Verification items for the finished model (mm, model axes). Face numbers are marked on the shaded views. A direction names the side the tool comes from. Round coordinates to 2 decimals unless told otherwise and drop trailing zeros. Write each loop counter-clockwise with the first axis right and the second up, starting at its lowest first coordinate (ties: lowest second). Pieces come first, ordered by that corner, then holes. Notation, with made-up numbers: (57, 87.25) - (109, 87.25) arc R33 cw to (109, 115.25) - close; hole circle Ø4 at (19, -5.5). An arc over 180 degrees is marked (long way). Answer as a JSON object with one key per item and string values. Group by question number.
1) Section check A-A (y = 30.5). Enter the section's corners in (x, z), then the cut area to 3 significant figures.
2) Section check D-D (x = -34.5). Enter the section's corners in (y, z).
3) Section check B-B (x = 8.5). Enter the section's corners in (y, z), then the cut area to 3 significant figures.
4) Section check C-C (z = 19). Enter the section's corners in (x, y), then the cut area to 3 significant figures.
5) Go/stop test with flat-tipped pins: pin 1 Ø4 at (y, z) = (124, 94) entering from +X; pin 2 Ø6.5 at (x, z) = (30, 95.5) entering from -Y; pin 3 Ø1.8 at (x, z) = (-25, 44.5) entering from +Y. Record where each tip stops, or that it passes through.
6) Mould release check, pull along X, two halves, no side actions. Record for the marked faces 4, 5 and 6: +X half, -X half, draft (parallel to the pull), parting line (faces both ways), or undercut.
7) Thickness scan on line 1 (Y direction, x = 19.5, z = 26.5); line 2 (Y direction, x = 46, z = 22); line 3 (Z direction, x = 13.5, y = 10). Record the ranges inside material, lowest first.
8) Set-up check for the marked faces 1, 2 and 3: record each of +Z, -Z, +X, -X, +Y, -Y from which the full face is reachable in a straight line by a thin tool's end or side.
Autodesk Inventor part; units mm, degrees
ref_plane "Work Plane1" through (-48, 65, 2) normal (0, -1, 0) x (1, 0, 0)
ref_plane "Work Plane3" through (-48, 165, 5) normal (0, 1, 0) x (1, 0, 0)
ref_plane "Work Plane2" through (-48, 165, 5) normal (0, 1, 0) x (1, 0, 0)
sketch "Sketch2" plane through (0, 0, 0) normal (0, 0, 1) x (1, 0, 0)
  line L0 (0, 0) -> (70, 0)
  line L1 (70, 0) -> (70, 165)
  line L2 (70, 165) -> (0, 165)
  line L3 (0, 165) -> (0, 0)
  dimension "d0" = 165
  dimension "d1" = 70
extrude "Extrusion1" add sketch "Sketch2" along normal blind 90
sketch "Sketch6" plane through (0, 0, 0) normal (-1, 0, 0) x (0, 0, 1)
  line L0 (90, 0) -> (90, 165)
  line L1 (0, 0) -> (0, 165)
  line L2 (90, 165) -> (0, 165)
  line L3 (0, 165) -> (0, 65)
  line L4 (0, 65) -> (90, 65)
  line L5 (90, 65) -> (90, 165)
  dimension "d8" = 100
extrude "Extrusion3" add sketch "Sketch6" along normal blind 50
sketch "Sketch7" plane through (0, 65, 0) normal (0, -1, 0) x (1, 0, 0)
  line L0 (70, 90) -> (-50, 90)
  line L1 (0, 0) -> (0, 90)
  line L2 (-50, 90) -> (0, 90)
  line L3 (0, 90) -> (0, 38)
  line L4 (0, 38) -> (-50, 38)
  line L5 (-50, 38) -> (-50, 90)
  dimension "d11" = 52
extrude "Extrusion4" add sketch "Sketch7" along normal blind 75
sketch "Sketch8" plane through (0, 65, 38) normal (0, 0, -1) x (-1, 0, 0)
  line L0 (0, 0) -> (50, 0)
  line L1 (50, 0) -> (29, 0)
  line L2 (29, 0) -> (29, -45)
  line L3 (29, -45) -> (50, -45)
  line L4 (50, -45) -> (50, 0)
  point P0 (0, -65)
  point P1 (29, 0)
  dimension "d14" = 21
  dimension "d15" = 45
extrude "Extrusion5" add sketch "Sketch8" along normal blind 25
sketch "Sketch9" plane through (0, 0, 90) normal (0, 0, 1) x (1, 0, 0)
  line L0 (70, 165) -> (-50, 165)
  line L1 (-50, 165) -> (70, 165)
  line L2 (70, 165) -> (10, 165)
  line L3 (10, 70) -> (57.5, 70)
  line L4 (57.5, 70) -> (-37.5, 70)
  line L5 (-37.5, 70) -> (-37.5, 165)
  line L6 (57.5, 70) -> (57.5, 165)
  point P0 (0, 0)
  dimension "d20" = 95
  dimension "d21" = 95
extrude "Extrusion6" add sketch "Sketch9" along normal blind 8
ref_plane "Work Plane1" through (-48, 65, 2) normal (0, -1, 0) x (1, 0, 0)
sketch "Sketch10" plane through (-48, 65, 2) normal (0, -1, 0) x (1, 0, 0)
  line L0 (21, 34) -> (46, 34)
  line L1 (33.5, 34) -> (33.5, 0)
  line L2 (46, 0) -> (0, 0)
  circle A0 centre (33.5, 17) radius 12.5
  point P0 (48, -2)
extrude "Extrusion7" add sketch "Sketch10" along normal blind 70
ref_plane "Work Plane3" through (-48, 165, 5) normal (0, 1, 0) x (1, 0, 0)
sketch "Sketch11" plane through (-48, 165, 5) normal (0, 1, 0) x (1, 0, 0)
  line L0 (113, 0) -> (113, -80)
  line L1 (0, -80) -> (0, 0)
  circle A0 centre (56.5, -40) radius 21
  point P0 (48, 5)
  dimension "d29" = 42
extrude "Extrusion8" add sketch "Sketch11" along normal blind 6
ref_plane "Work Plane2" through (-48, 165, 5) normal (0, 1, 0) x (1, 0, 0)
sketch "Sketch12" plane through (-48, 165, 5) normal (0, 1, 0) x (1, 0, 0)
  circle A0 centre (56.5, -40) radius 21
  line L0 (35.5, -40) -> (26.5, -40)
  circle A1 centre (23.5, -40) radius 3
  point P0 (48, 5)
  dimension "d32" = 9
extrude "Extrusion9" add sketch "Sketch12" along normal blind 7 contours A1
sketch "Sketch13" plane through (8.5, 171, 45) normal (0, 1, 0) x (1, 0, 0)
  circle A0 centre (0, 0) radius 22.5
  arc A1 (21.4111, -6.9148) -> (21.4111, 6.9148) centre (22.5, 0) ccw
  point P0 (-8.5, 45)
  dimension "d37" = 45
  dimension "d38" = 14
extrude "Extrusion10" add sketch "Sketch13" along normal mid plane 6 contours A0
extrude "Extrusion11" add sketch "Sketch13" along normal blind 2 contours A0 A1
fillet "Fillet3" radius 10 4 edges at (-50, 115, 0) (70, 82.5, 0) (70, 82.5, 90) (-50, 77.5, 90)
properties part number "windshield washer"
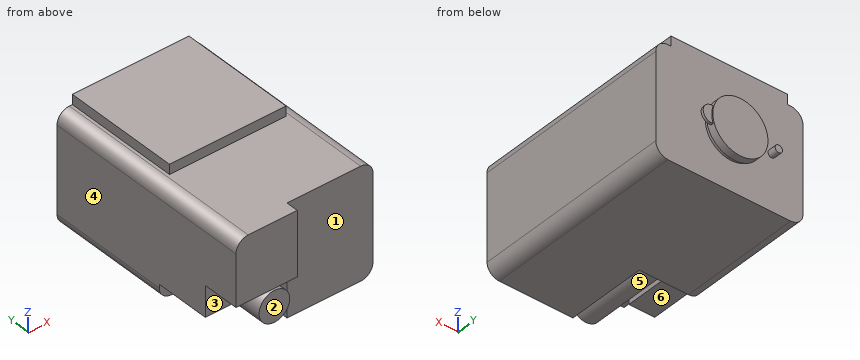
Returned:
{
 "1": {"outline": "(-50, 13) - (-29, 13) - (-29, 38) - (0, 38) - (0, 0) - (60, 0) arc R10 ccw to (70, 10) - (70, 80) arc R10 ccw to (60, 90) - (-40, 90) arc R10 ccw to (-50, 80) - close; circle Ø25 at (-14.5, 19)", "area": "9,850 mm2"},
 "2": {"outline": "(-10, 38) - (20, 38) - (20, 13) - (65, 13) - (65, 0) - (165, 0) - (165, 98) - (70, 98) - (70, 90) - (-10, 90) - close"},
 "3": {"outline": "(0, 0) - (165, 0) - (165, 24) - (168, 24) - (168, 22.5) - (174, 22.5) - (174, 67.5) - (168, 67.5) - (168, 66) - (165, 66) - (165, 98) - (70, 98) - (70, 90) - (0, 90) - close", "area": "16,000 mm2"},
 "4": {"outline": "(-50, 20) - (-29, 20) - (-29, 65) - (-27, 65) - (-27, -5) - (-2, -5) - (-2, 65) - (0, 65) - (0, 0) - (70, 0) - (70, 165) - (-50, 165) - close", "area": "19,200 mm2"},
 "5": {"pin 1": "x = 57.5", "pin 2": "y = 70", "pin 3": "y = 172"},
 "6": {"face 4": "-X half", "face 5": "undercut", "face 6": "draft"},
 "7": {"line 1": "0 to 165, 168 to 174", "line 2": "0 to 165", "line 3": "0 to 90"},
 "8": {"face 1": "+Z, -Z, +X, -Y", "face 2": "-Z, +X, -X, -Y", "face 3": "-Z, -X, -Y"}
}
